from build123d import *

# Parameters (mm, degrees)
F0_W     = 60
F0_H     = 60
F1_DEPTH = 30
F2_W     = 40
F2_H     = 40
F3_DEPTH = 30
F4_W     = 40
F4_H     = 20
F5_DEPTH = 60
F6_W     = 40
F6_H     = 20
F7_DEPTH = 60
F8_W     = 5.5
F8_H     = 5.5
F9_DEPTH = 20
F10_R    = 3


with BuildPart() as f1:
    # F0 (on Top) → F1 (new body)
    with BuildSketch(Plane.XY):
        Rectangle(F0_W, F0_H)
    extrude(amount=F1_DEPTH)

    # F2 (on face) → F3 (cut)
    with BuildSketch(Plane.XY.offset(30)):
        Rectangle(F2_W, F2_H)
    extrude(amount=-F3_DEPTH, mode=Mode.SUBTRACT)

    # F4 (on face) → F5 (cut)
    with BuildSketch(Plane.YZ.offset(30)):
        with Locations((0, 20)):
            Rectangle(F4_W, F4_H)
    extrude(amount=-F5_DEPTH, mode=Mode.SUBTRACT)

    # F6 (on face) → F7 (cut)
    with BuildSketch(Plane.XZ.offset(30)):
        with Locations((0, 20)):
            Rectangle(F6_W, F6_H)
    extrude(amount=-F7_DEPTH, mode=Mode.SUBTRACT)

    # F8 (on face) → F9 (cut)
    with BuildSketch(Plane.XY.offset(30)):
        with Locations((-22.75, -22.75)):
            Rectangle(F8_W, F8_H)
    extrude(amount=-F9_DEPTH, mode=Mode.SUBTRACT)

    # F10
    f10_edges = [f1.edges().sort_by_distance(p)[0] for p in [
        (30, 30, 15),
        (0, 30, 0),
        (-30, 30, 15),
        (30, -30, 15),
        (-30, -30, 15),
        (0, -30, 0),
        (-30, 0, 0),
        (30, 0, 0),
    ]]
    fillet(f10_edges, radius=F10_R)


solid = f1.part
Can you work these out from the model? Positions are in its coordinate system, mm. A direction names the side the tool comes from. Give positions to 0.01 mm unless a question says otherwise; leave off trailing zeros. Order: outer loops, then holes, each group sorted by start corner. A loop starts at its lowest first (then second) coordinate and runs counter-clockwise, first axis right, second up. Notation, with made-up numbers: M 66,34 L 95,34 A34 ccw 95,73 Z; hole C 5.5,68 d10. An arc over 180 degrees is marked long. Use one line per item in the form item = value. Start each with the question number.
Item 1: Will these pins go through, and if not, where does the flat tip stop? pin 1 Ø1 at (x, y) = (-22, 6) entering from -Z; pin 2 Ø8 at (x, y) = (27.5, -3) entering from +Z; pin 3 Ø1.3 at (y, z) = (-29, 19) entering from +X; pin 4 Ø2 at (x, z) = (-28.5, 20.5) entering from +Y.
Item 2: If we section it at C-C (y = -6): Write out the boundary of the cut face in (x, z).
Item 3: If we section it at B-B (z = 4): Write out the boundary of the cut face in (x, y), then the cut area to 3 significant figures.
Item 4: If we section it at A-A (z = 22.5): Write out the boundary of the cut face in (x, y), then the cut area to 3 significant figures.
Item 5: For faces 5 (the flat face through (-20, 0, 5)), 6 (the flat face through (20, 25, 20)), 7 (the flat face through (-30, 0, 7)), 8 (the flat face through (-25, 20, 20)), which set-ups out of +Z, -Z, +X, -X, +Y, -Y let a thin tool reach every point of the face, with its end or its side?
Item 6: If I drill on line 1 along X through (y, z) = (-24, 23.25); line 2 along X through (y, z) = (-26, 28.5), over which ranges is the centre line in solid material (lowest first)?
Item 7: We'd pull the mould along X, two halves only. Please class faces 1 (the flat face through (-20, 25, 20)), 2 (the flat face through (-28, -20, 20)), 3 (the flat face through (-23, -25.5, 20)), 4 (the cylindrical face through (29.1, -29.14, 16.69)): +X half, -X half, draft (parallel to the pull), parting line (faces both ways), or undercut.
Outcome:
q1.pin_1 = 0
q1.pin_2 = 10
q1.pin_3 = 29.68
q1.pin_4 = 29.96
q2.outline = M -30,3 A3 ccw -27,0 L -20,0 L -20,10 L -30,10 Z; M 20,0 L 27,0 A3 ccw 30,3 L 30,10 L 20,10 Z
q3.outline = M -30,-27 A3 ccw -27,-30 L 27,-30 A3 ccw 30,-27 L 30,27 A3 ccw 27,30 L -27,30 A3 ccw -30,27 Z; hole M -20,-20 L 20,-20 L 20,20 L -20,20 Z
q3.area = 1,990 mm2
q4.outline = M -30,-27 A3 ccw -27,-30 L -20,-30 L -20,-25.5 L -25.5,-25.5 L -25.5,-20 L -30,-20 Z; M -30,20 L -20,20 L -20,30 L -27,30 A3 ccw -30,27 Z; M 20,-30 L 27,-30 A3 ccw 30,-27 L 30,-20 L 20,-20 Z; M 20,20 L 30,20 L 30,27 A3 ccw 27,30 L 20,30 Z
q4.area = 362 mm2
q5.face_5 = +Z, -Z
q5.face_6 = +Z, +Y, -Y
q5.face_7 = +Z, -Z, -X, +Y, -Y
q5.face_8 = +Z, +X, -X
q6.line_1 = -30 to -25.5, 20 to 30
q6.line_2 = -30 to -20, 20 to 30
q7.face_1 = undercut
q7.face_2 = draft
q7.face_3 = undercut
q7.face_4 = +X half
